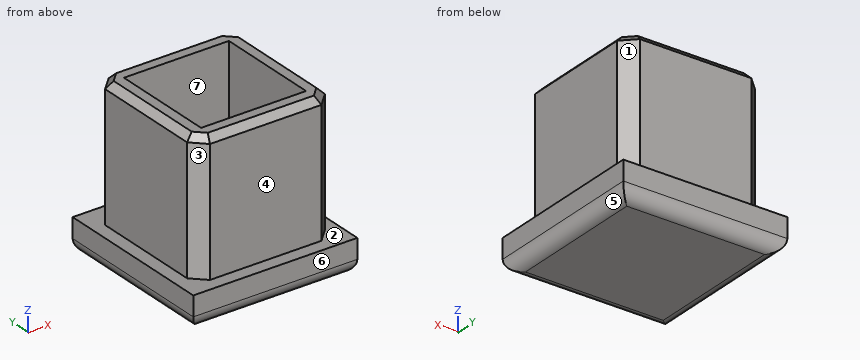
from build123d import *

# Parameters (mm, degrees)
SKETCH_W        = 25
SKETCH_H        = 25
PAD_DEPTH       = 25
SKETCH001_W     = 25
SKETCH001_H     = 25
SKETCH001_W_2   = 21
SKETCH001_H_2   = 21
POCKET_DEPTH    = 20
SKETCH002_W     = 16
SKETCH002_H     = 16
POCKET001_DEPTH = 22
CHAMFER_SIZE    = 2
FILLET_R        = 2
CHAMFER001_SIZE = 1


with BuildPart() as part:
    # Sketch → Pad (new body)
    with BuildSketch(Plane.XY):
        with Locations((12.5, 12.5)):
            Rectangle(SKETCH_W, SKETCH_H)
    extrude(amount=PAD_DEPTH)

    # Sketch001 (on Face6 of Pad) → Pocket (cut)
    with BuildSketch(Plane.XY.offset(25)):
        with Locations((12.5, 12.5)):
            Rectangle(SKETCH001_W, SKETCH001_H)
        with Locations((12.5, 12.5)):
            Rectangle(SKETCH001_W_2, SKETCH001_H_2, mode=Mode.SUBTRACT)
    extrude(amount=-POCKET_DEPTH, mode=Mode.SUBTRACT)

    # Sketch002 (on Face11 of Pocket) → Pocket001 (cut)
    with BuildSketch(Plane.XY.offset(25)):
        with Locations((12.5, 12.5)):
            Rectangle(SKETCH002_W, SKETCH002_H)
    extrude(amount=-POCKET001_DEPTH, mode=Mode.SUBTRACT)

    # Chamfer
    chamfer_edges = [part.edges().sort_by_distance(p)[0] for p in [
        (2, 2, 15),
        (23, 2, 15),
        (2, 23, 15),
        (23, 23, 15),
    ]]
    chamfer(chamfer_edges, length=CHAMFER_SIZE)

    # Fillet
    fillet_edges = [part.edges().sort_by_distance(p)[0] for p in [
        (12.5, 0, 0),
        (25, 12.5, 0),
        (12.5, 25, 0),
        (0, 12.5, 0),
    ]]
    fillet(fillet_edges, radius=FILLET_R)

    # Chamfer001
    chamfer001_edges = [part.edges().sort_by_distance(p)[0] for p in [
        (23, 12.5, 25),
        (22, 3, 25),
        (12.5, 2, 25),
        (3, 3, 25),
        (2, 12.5, 25),
        (3, 22, 25),
        (12.5, 23, 25),
        (22, 22, 25),
    ]]
    chamfer(chamfer001_edges, length=CHAMFER001_SIZE)


solid = part.part
Design review of the part built by this model. Coordinates are the model's own, in mm. Face numbers are marked on the shaded views. A direction names the side the tool comes from. Coordinates: 2 decimals unless noted, no trailing zeros. Order: outer loops, then holes, each group sorted by start corner. A loop starts at its lowest first (then second) coordinate and runs counter-clockwise, first axis right, second up.
Item 1: The part is to be moulded in two halves that separate along X. For the marked faces 5, 6 and 7, say which applies: pulls with the +X half, pulls with the -X half, needs draft (parallel to the pull), parting line crosses it, or undercut.
Item 2: Take a section at D-D, the plane z = 3.5. Write out the cut boundary in (x, y), then the cut area to 3 significant figures.
Item 3: For line 1 (X direction, y = 8, z = 4.75); line 2 (Y direction, x = 17.5, z = 8.5), list the stretches that pass through material, from the lowest coordinate up.
Item 4: Take a section at B-B, the plane y = 6.75. Write out the cut boundary in (x, z).
Item 5: For the marked faces 1, 2, 3 and 4, list the 3-axis set-ups (+Z, -Z, +X, -X, +Y, -Y) from which the entire face can be reached by the end or side of a thin tool; tool diameter is ignored.
Item 6: Take a section at A-A, the plane z = 17.25. Write out the cut boundary in (x, y), then the cut area to 3 significant figures.
Item 7: For pin 1 Ø13.5 at (y, z) = (15.5, 17) entering from +X; pin 2 Ø8 at (x, z) = (8.5, 15.5) entering from +Y; pin 3 Ø12.5 at (x, y) = (17.5, 12.5) entering from +Z; pin 4 Ø10 at (y, z) = (15.5, 16) entering from -X, all flat-tipped, find the tip position at first contact; note any pin that passes through.
The answers:
1. face 5: pulls with the +X half
1. face 6: needs draft
1. face 7: undercut
2. outline: (0, 0) - (25, 0) - (25, 25) - (0, 25) - close; hole (4.5, 4.5) - (20.5, 4.5) - (20.5, 20.5) - (4.5, 20.5) - close
2. area: 369 mm2
3. line 1: x = 0 to 4.5, 20.5 to 25
3. line 2: y = 2 to 4.5, 20.5 to 23
4. outline: (0, 2) arc R2 ccw to (2, 0) - (23, 0) arc R2 ccw to (25, 2) - (25, 5) - (23, 5) - (23, 24) - (22, 25) - (20.5, 25) - (20.5, 3) - (4.5, 3) - (4.5, 25) - (3, 25) - (2, 24) - (2, 5) - (0, 5) - close
5. face 1: +Z, +X, +Y
5. face 2: +Z
5. face 3: +Z, -X, -Y
5. face 4: +Z, +X, -X, -Y
6. outline: (2, 4) - (4, 2) - (21, 2) - (23, 4) - (23, 21) - (21, 23) - (4, 23) - (2, 21) - close; hole (4.5, 4.5) - (20.5, 4.5) - (20.5, 20.5) - (4.5, 20.5) - close
6. area: 177 mm2
7. pin 1: stops at x = 23
7. pin 2: stops at y = 23
7. pin 3: stops at z = 25
7. pin 4: stops at x = 2
